Check sheet for the modelled part. Datum: model origin and axes. Units: mm. Face numbers are marked on the shaded views. A direction names the side the tool comes from. Give positions to 0.01 mm unless a question says otherwise; leave off trailing zeros. Order: outer loops, then holes, each group sorted by start corner. A loop starts at its lowest first (then second) coordinate and runs counter-clockwise, first axis right, second up. Notation, with made-up numbers: (-2, -4.75) -> (45, -4.75) arc R7 cw to (45, -0.75) -> close; hole circle Ø4 at (-23.75, -2). An arc over 180 degrees is marked (long way). Write each question's results on one line, items separated by ' | '.
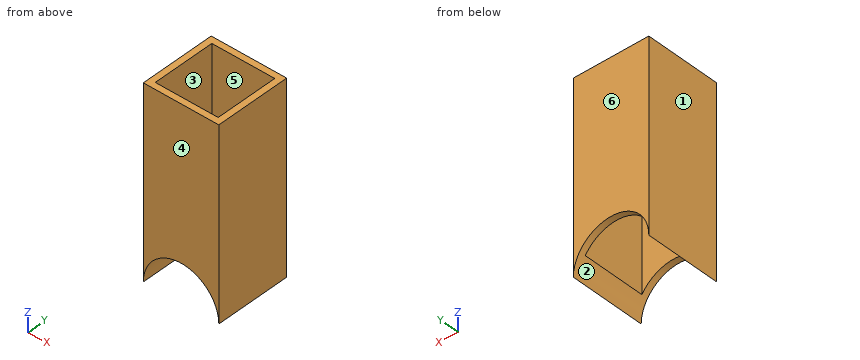
from build123d import *

# Parameters (mm, degrees)
SKETCH1_W           = 30
SKETCH1_H           = 30
SKETCH1_W_2         = 25
SKETCH1_H_2         = 25
BOSS_EXTRUDE1_DEPTH = 75
SKETCH2_R           = 15
CUT_EXTRUDE1_DEPTH  = 83.158383626


with BuildPart() as part:
    # Sketch1 → Boss-Extrude1 (new body)
    with BuildSketch(Plane.XY):
        Rectangle(SKETCH1_W, SKETCH1_H)
        Rectangle(SKETCH1_W_2, SKETCH1_H_2, mode=Mode.SUBTRACT)
    extrude(amount=BOSS_EXTRUDE1_DEPTH)

    # Sketch2 → Cut-Extrude1 (cut, through all)
    with BuildSketch(Plane.XZ.offset(15)):
        Circle(SKETCH2_R)
    extrude(amount=-CUT_EXTRUDE1_DEPTH, mode=Mode.SUBTRACT)


solid = part.part
1. Section check A-A on x = 0. Record the cut outline in (y, z).
Verdict:
outline: (-15, 15) -> (-12.5, 15) -> (-12.5, 75) -> (-15, 75) -> close; (12.5, 15) -> (15, 15) -> (15, 75) -> (12.5, 75) -> close
2. Access from +Z, -Z, +X, -X, +Y, -Y to the whole of each face (thin tool, end or side, straight path). Record for the marked faces 5 and 6.
Verdict:
face 5: +Z, -Z | face 6: +Z, -Z, +X, -X, +Y
3. Mould release check, pull along X, two halves, no side actions. Record for the marked faces 1, 2, 3 and 4: +X half, -X half, draft (parallel to the pull), parting line (faces both ways), or undercut.
Verdict:
face 1: -X half | face 2: undercut | face 3: undercut | face 4: draft
4. Gauge pin test, flat end, axial feed: pin 1 Ø6 at (x, y) = (0, -11) entering from -Z. Record the tip position at first contact, or that the pin passes through.
Verdict:
pin 1: stops at z = 14.77
5. Material ranges on probe 1 along X at (y, z) = (4.5, 52); probe 2 along Z at (x, y) = (0.75, -13), recorded low to high. Write a range as from..to.
Verdict:
probe 1: x = -15..-12.5, 12.5..15 | probe 2: z = 14.98..75
6. Section check B-B on y = -0.5. Record the cut outline in (x, z), then the cut area to 3 significant figures.
Verdict:
outline: (-15, 0) arc R15 cw to (-12.5, 8.29) -> (-12.5, 75) -> (-15, 75) -> close; (12.5, 8.29) arc R15 cw to (15, 0) -> (15, 75) -> (12.5, 75) -> close | area: 347 mm^2
7. Section check D-D on y = 13.25. Record the cut outline in (x, z), then the cut area to 3 significant figures.
Verdict:
outline: (-15, 0) arc R15 cw to (15, 0) -> (15, 75) -> (-15, 75) -> close | area: 1,900 mm^2
8. Section check C-C on z = 16. Record the cut outline in (x, y).
Verdict:
outline: (-15, -15) -> (15, -15) -> (15, 15) -> (-15, 15) -> close; hole (-12.5, -12.5) -> (12.5, -12.5) -> (12.5, 12.5) -> (-12.5, 12.5) -> close
